```python
from build123d import *

# Parameters (mm, degrees)
SKETCH1_W           = 72
SKETCH1_H           = 55
BOSS_EXTRUDE1_DEPTH = 4
FILLET3_R           = 5
FILLET4_R           = 5
CUT_EXTRUDE1_DEPTH  = 0.25
SKETCH3_W           = 62
SKETCH3_H           = 46
SKETCH3_W_2         = 60
SKETCH3_H_2         = 44
BOSS_EXTRUDE2_DEPTH = 4
SKETCH4_W           = 65
SKETCH4_H           = 49
SKETCH4_W_2         = 60
SKETCH4_H_2         = 44
BOSS_EXTRUDE3_DEPTH = 1
FILLET2_R           = 2
BOSS_EXTRUDE4_DEPTH = 0.5
BOSS_EXTRUDE5_DEPTH = 26
SKETCH7_R           = 1
BOSS_EXTRUDE6_DEPTH = 29.5
CUT_EXTRUDE2_DEPTH  = 15
CHAMFER1_SIZE       = 0.5


with BuildPart() as part:
    # Sketch1 → Boss-Extrude1 (new body)
    with BuildSketch(Plane.XY):
        Rectangle(SKETCH1_W, SKETCH1_H)
    extrude(amount=BOSS_EXTRUDE1_DEPTH)

    # Fillet3
    fillet3_edges = [part.edges().sort_by_distance(p)[0] for p in [
        (36, -27.5, 2),
        (-36, -27.5, 2),
        (-36, 27.5, 2),
        (36, 27.5, 2),
    ]]
    fillet(fillet3_edges, radius=FILLET3_R)

    # Fillet4
    # the kernel refuses this fillet: 5 mm, written as the material it takes off along each edge
    with BuildSketch(Plane(origin=(31, 22.5, 4), x_dir=(1, 0, 0), z_dir=(0, -1, 0))) as fillet4_piece_1:
        with BuildLine():
            CenterArc((0.101020514, -5), FILLET4_R, 11.536959033, 78.463040967)
            Line((5, -4), (5.09797959, -3.98))
            ThreePointArc((5.09797959, -3.98), (5.1, -2), (5.1, 0))
            Line((5.1, 0), (5, 0.1))
            Line((5, 0.1), (0.101020514, 0.1))
            Line((0.101020514, 0.1), (0.101020514, 0))
        make_face()
    revolve(axis=Axis((31, 22.5, 4), (0, 0, 1)), revolution_arc=90, mode=Mode.SUBTRACT)
    with BuildSketch(Plane(origin=(36, -22.5, 4), x_dir=(-1, 0, 0), z_dir=(0, 1, 0)), Plane(origin=(-36, 22.5, 4), x_dir=(1, 0, 0), z_dir=(0, -1, 0))) as fillet4_piece_2:
        with BuildLine():
            CenterArc((4.898979486, -5), FILLET4_R, 90, 78.463040967)
            Line((0, -4), (-0.09797959, -3.98))
            ThreePointArc((-0.09797959, -3.98), (-0.1, -2), (-0.1, 0))
            Line((-0.1, 0), (0, 0.1))
            Line((0, 0.1), (4.898979486, 0.1))
            Line((4.898979486, 0.1), (4.898979486, 0))
        make_face()
    extrude(amount=45, mode=Mode.SUBTRACT)
    with BuildSketch(Plane(origin=(31, -22.5, 4), x_dir=(0, -1, 0), z_dir=(-1, 0, 0))) as fillet4_piece_3:
        with BuildLine():
            CenterArc((0.101020514, -5), FILLET4_R, 11.536959033, 78.463040967)
            Line((0.101020514, 0), (0.101020514, 0.1))
            Line((0.101020514, 0.1), (5, 0.1))
            Line((5, 0.1), (5.1, 0))
            ThreePointArc((5.1, 0), (5.1, -2), (5.09797959, -3.98))
            Line((5.09797959, -3.98), (5, -4))
        make_face()
    revolve(axis=Axis((31, -22.5, 4), (0, 0, 1)), revolution_arc=90, mode=Mode.SUBTRACT)
    with BuildSketch(Plane(origin=(-31, -27.5, 4), x_dir=(0, 1.564970375511121e-12, -1.0), z_dir=(1, 0, 0))) as fillet4_piece_4:
        with BuildLine():
            CenterArc((5, 4.898979486), FILLET4_R, 180, 78.463040967)
            Line((0, 4.898979486), (-0.1, 4.898979486))
            Line((-0.1, 4.898979486), (-0.1, 0))
            Line((-0.1, 0), (0, -0.1))
            ThreePointArc((0, -0.1), (2, -0.1), (3.98, -0.09797959))
            Line((3.98, -0.09797959), (4, 0))
        make_face()
    extrude(amount=62, mode=Mode.SUBTRACT)
    with BuildSketch(Plane(origin=(-31, -22.5, 4), x_dir=(0, -1, 0), z_dir=(1, 0, 0))) as fillet4_piece_5:
        with BuildLine():
            CenterArc((0.101020514, 5), FILLET4_R, 270, 78.463040967)
            Line((0.101020514, 0), (0.101020514, -0.1))
            Line((0.101020514, -0.1), (5, -0.1))
            Line((5, -0.1), (5.1, 0))
            ThreePointArc((5.1, 0), (5.1, 2), (5.09797959, 3.98))
            Line((5.09797959, 3.98), (5, 4))
        make_face()
    revolve(axis=Axis((-31, -22.5, 4), (0, 0, -1)), revolution_arc=90, mode=Mode.SUBTRACT)
    with BuildSketch(Plane(origin=(-31, 22.5, 4), x_dir=(0, 1, 0), z_dir=(1, 0, 0))) as fillet4_piece_6:
        with BuildLine():
            CenterArc((0.101020514, -5), FILLET4_R, 11.536959033, 78.463040967)
            Line((5, -4), (5.09797959, -3.98))
            ThreePointArc((5.09797959, -3.98), (5.1, -2), (5.1, 0))
            Line((5.1, 0), (5, 0.1))
            Line((5, 0.1), (0.101020514, 0.1))
            Line((0.101020514, 0.1), (0.101020514, 0))
        make_face()
    revolve(axis=Axis((-31, 22.5, 4), (0, 0, 1)), revolution_arc=90, mode=Mode.SUBTRACT)
    with BuildSketch(Plane(origin=(31, 27.5, 4), x_dir=(0, -1, 0), z_dir=(-1, 0, 0))) as fillet4_piece_7:
        with BuildLine():
            CenterArc((4.898979486, -5), FILLET4_R, 90, 78.463040967)
            Line((0, -4), (-0.09797959, -3.98))
            ThreePointArc((-0.09797959, -3.98), (-0.1, -2), (-0.1, 0))
            Line((-0.1, 0), (0, 0.1))
            Line((0, 0.1), (4.898979486, 0.1))
            Line((4.898979486, 0.1), (4.898979486, 0))
        make_face()
    extrude(amount=62, mode=Mode.SUBTRACT)

    # Sketch2 → Cut-Extrude1 (cut)
    with BuildSketch(Plane.XY.offset(4)):
        with BuildLine():
            Line((31.101020514, -22.5), (31.101020514, 22.5))
            ThreePointArc((31.101020514, 22.5), (31.071432291, 22.571432291), (31, 22.601020514))
            Line((31, 22.601020514), (-31, 22.601020514))
            ThreePointArc((-31, 22.601020514), (-31.071432291, 22.571432291), (-31.101020514, 22.5))
            Line((-31.101020514, 22.5), (-31.101020514, -22.5))
            ThreePointArc((-31.101020514, -22.5), (-31.071432291, -22.571432291), (-31, -22.601020514))
            Line((-31, -22.601020514), (31, -22.601020514))
            ThreePointArc((31, -22.601020514), (31.071432291, -22.571432291), (31.101020514, -22.5))
        make_face()
    extrude(amount=-CUT_EXTRUDE1_DEPTH, mode=Mode.SUBTRACT)

    # Sketch3 → Boss-Extrude2 (add)
    with BuildSketch(Plane(origin=(0, 0, 0), x_dir=(-1, 0, 0), z_dir=(0, 0, -1))):
        Rectangle(SKETCH3_W, SKETCH3_H)
        Rectangle(SKETCH3_W_2, SKETCH3_H_2, mode=Mode.SUBTRACT)
    extrude(amount=BOSS_EXTRUDE2_DEPTH)

    # Sketch4 → Boss-Extrude3 (add)
    with BuildSketch(Plane(origin=(0, 0, -4), x_dir=(-1, 0, 0), z_dir=(0, 0, -1))):
        Rectangle(SKETCH4_W, SKETCH4_H)
        Rectangle(SKETCH4_W_2, SKETCH4_H_2, mode=Mode.SUBTRACT)
    extrude(amount=-BOSS_EXTRUDE3_DEPTH)

    # Fillet2
    fillet2_edges = [part.edges().sort_by_distance(p)[0] for p in [
        (31, 23, -1.5),
        (-31, 23, -1.5),
        (-31, -23, -1.5),
        (31, -23, -1.5),
        (32.5, 24.5, -3.5),
        (-32.5, 24.5, -3.5),
        (-32.5, -24.5, -3.5),
        (32.5, -24.5, -3.5),
        (-30, 22, -2),
        (30, 22, -2),
        (30, -22, -2),
        (-30, -22, -2),
    ]]
    fillet(fillet2_edges, radius=FILLET2_R)

    # Sketch5 → Boss-Extrude4 (add)
    with BuildSketch(Plane(origin=(0, 0, 0), x_dir=(-1, 0, 0), z_dir=(0, 0, -1))):
        with BuildLine():
            Line((-15, 7), (15, 7))
            ThreePointArc((15, 7), (22, 0), (15, -7))
            Line((15, -7), (-15, -7))
            ThreePointArc((-15, -7), (-22, 0), (-15, 7))
        make_face()
        with BuildLine():
            Line((-15, 5.5), (15, 5.5))
            ThreePointArc((15, 5.5), (20.5, 0), (15, -5.5))
            Line((15, -5.5), (-15, -5.5))
            ThreePointArc((-15, -5.5), (-20.5, 0), (-15, 5.5))
        make_face(mode=Mode.SUBTRACT)
    extrude(amount=BOSS_EXTRUDE4_DEPTH)

    # Sketch6 → Boss-Extrude5 (add, symmetric)
    with BuildSketch(Plane(origin=(0, 0, 0), x_dir=(0, 0, -1), z_dir=(1, 0, 0))):
        with BuildLine():
            Line((0, 27.5), (0, 29))
            ThreePointArc((0, 29), (-0.146446609, 29.353553391), (-0.5, 29.5))
            Line((-0.5, 29.5), (-4.5, 29.5))
            ThreePointArc((-4.5, 29.5), (-4.853553391, 29.353553391), (-5, 29))
            Line((-5, 29), (-5, 28))
            ThreePointArc((-5, 28), (-4.853553391, 27.646446609), (-4.5, 27.5))
            Line((-4.5, 27.5), (-3.707106781, 27.5))
            ThreePointArc((-3.707106781, 27.5), (-3.515765065, 27.461939766), (-3.353553391, 27.353553391))
            Line((-3.353553391, 27.353553391), (-1.948480403, 25.948480403))
            Line((-1.948480403, 25.948480403), (0, 25.948480403))
            Line((0, 25.948480403), (0, 27.5))
        make_face()
    extrude(amount=BOSS_EXTRUDE5_DEPTH, both=True)

    # Sketch7 → Boss-Extrude6 (add, symmetric)
    with BuildSketch(Plane(origin=(0, 0, 0), x_dir=(0, 0, -1), z_dir=(1, 0, 0))):
        with BuildLine():
            Line((-2.16812286, -31.451484043), (-3.76812286, -28.00017482))
            ThreePointArc((-3.76812286, -28.00017482), (-3.941342576, -27.487064649), (-4, -26.948690777))
            Line((-4, -26.948690777), (-4, -22.601020514))
            ThreePointArc((-4, -22.601020514), (-2.872983346, -25.763298175), (0, -27.5))
            Line((0, -27.5), (0.1, -27.9))
            ThreePointArc((0.1, -27.9), (2.206977706, -31.745602076), (-2.16812286, -31.451484043))
        make_face()
        with Locations((0.1, -30.4)):
            Circle(SKETCH7_R, mode=Mode.SUBTRACT)
    extrude(amount=BOSS_EXTRUDE6_DEPTH, both=True)

    # Sketch8 → Cut-Extrude2 (cut, symmetric)
    with BuildSketch(Plane(origin=(0, 0, 0), x_dir=(0, 0, -1), z_dir=(1, 0, 0))):
        with BuildLine():
            Line((0.1, -27.9), (0, -27.5))
            ThreePointArc((0, -27.5), (-2.872983346, -25.763298175), (-4, -22.601020514))
            Line((-4, -22.601020514), (-4, -26.948690777))
            ThreePointArc((-4, -26.948690777), (-3.941342576, -27.487064649), (-3.76812286, -28.00017482))
            Line((-3.76812286, -28.00017482), (-2.16812286, -31.451484043))
            ThreePointArc((-2.16812286, -31.451484043), (2.206977706, -31.745602076), (0.1, -27.9))
        make_face()
    extrude(amount=CUT_EXTRUDE2_DEPTH, both=True, mode=Mode.SUBTRACT)

    # Chamfer1
    chamfer1_edges = [part.edges().sort_by_distance(p)[0] for p in [
        (-29.5, -30.4, 0.9),
        (29.5, -30.4, 0.9),
    ]]
    chamfer(chamfer1_edges, length=CHAMFER1_SIZE)


solid = part.part
```
Work out the finished part from the listing and answer in its coordinate system (mm). A direction names the side the tool comes from. Round coordinates to 2 decimals unless told otherwise and drop trailing zeros. Loops run counter-clockwise (first coordinate to the right, second up) from the corner with the lowest first, then second, coordinate; pieces in that order, holes last. Notation, with made-up numbers: M 76,59.5 L 106,59.5 A18 cw 106,79.5 Z; hole C 59,20 d8. An arc over 180 degrees is marked long. Use CSV: the item, a comma, the result in double quotes.
Q1. The mould has two halves that part along Z. Classify faces 5 (the flat face through (0, 0, 0)), 6 (the cylindrical face through (-20.5, 0.1, -0.2)), 7 (the cylindrical face through (30.43, 22.4, -1.52)): pulls with the +Z half, pulls with the -Z half, needs draft (parallel to the pull), parting line crosses it, or undercut.
Determined:
face 5,"pulls with the -Z half"
face 6,"needs draft"
face 7,"undercut"
Q2. Consider L1, parallel to X at y = 6, z = -2; L2, parallel to Y at x = 26, z = -2.25; L3, parallel to Y at x = 23, z = -0.5. Determine where each line is inside the solid, lowest interval first.
Determined:
L1,"-31 to -30, 30 to 31"
L2,"-31.68 to -29.12, -23 to -22, 22 to 23"
L3,"-32.87 to -31.32, -29.48 to -27.93, -23 to -22, 22 to 23"
Q3. Each of these flat-tipped pins is pushed along its axis until it touches: pin 1 (1.5 mm diameter, centred on x = 5, z = -2, fed in from -Y); pin 2 (7 mm diameter, centred on x = 8.5, y = -1.5, fed in from -Z); pin 3 (0.8 mm diameter, centred on y = 2, z = -3.5, fed in from +X). Where does it stop, or does it pass through?
Determined:
pin 1,"y = -23"
pin 2,"z = 0"
pin 3,"x = 32.5"
Q4. A tool of negligible diameter and unlimited length cuts with its end or side. For faces 1 (the flat face through (1, 25, 0)), 2 (the flat face through (15, -29, 1)), 3 (the cylindrical face through (20.5, -0.1, -0.2)), 4 (the cylindrical face through (-31.93, 23.9, -3.49)), from which of +Z, -Z, +X, -X, +Y, -Y can it reach the whole face along a straight path? Write none if from no direction.
Determined:
face 1,"none"
face 2,"+Z, -Y"
face 3,"-Z"
face 4,"-Z, -X, +Y"
Q5. Section C-C, the plane y = -30.4 is taken. Determine the outline of the cut face in (x, z), then the cut area to 3 significant figures.
Determined:
outline,"M -29.5,-2.6 L -15,-2.6 L -15,-1.1 L -29,-1.1 L -29.5,-1.6 Z; M -29.5,1.4 L -29,0.9 L -15,0.9 L -15,2.66 L -29.5,2.66 Z; M 15,-2.6 L 29.5,-2.6 L 29.5,-1.6 L 29,-1.1 L 15,-1.1 Z; M 15,0.9 L 29,0.9 L 29.5,1.4 L 29.5,2.66 L 15,2.66 Z"
area,"93.9 mm2"
Q6. Section A-A, the plane y = -12 is taken. Determine the outline of the cut face in (x, z).
Determined:
outline,"M -36,0 L -31,0 L -31,-3 L -32.5,-3 L -32.5,-4 L -30,-4 L -30,0 L 30,0 L 30,-4 L 32.5,-4 L 32.5,-3 L 31,-3 L 31,0 L 36,0 A5 ccw 31.1,4 L 31.1,3.75 L -31.1,3.75 L -31.1,4 A5 ccw Z"
